Model file for the job. Use its own axes, mm. A direction names the side the tool comes from. Coordinates: 2 decimals unless noted, no trailing zeros. Write each loop counter-clockwise with the first axis right and the second up, starting at its lowest first coordinate (ties: lowest second). Pieces come first, ordered by that corner, then holes. Notation, with made-up numbers: (-16, 42.5) -> (42, 42.5) arc R27 cw to (42, 72.5) -> close; hole circle Ø6 at (-14.75, -26). An arc over 180 degrees is marked (long way). Answer as a JSON object with one key per item and string values. Group by question number.
from build123d import *

# Parameters (mm, degrees)
F1_DEPTH = 50
F1_TAPER = 17
F2_R     = 1
F3_R     = 25
F4_DEPTH = 2


with BuildPart() as f1:
    # F0 (on Top) → F1 (new body)
    with BuildSketch(Plane.XY):
        with BuildLine():
            Line((52.6273290813, 55.3626765174), (-57.3726709187, 55.3626765174))
            ThreePointArc((-57.3726709187, 55.3626765174), (-71.5148065424, 49.5048121412), (-77.3726709187, 35.3626765174))
            Line((-77.3726709187, 35.3626765174), (-77.3726709187, 5.3626765174))
            ThreePointArc((-77.3726709187, 5.3626765174), (-71.5148065424, -8.7794591063), (-57.3726709187, -14.6373234826))
            Line((-57.3726709187, -14.6373234826), (52.6273290813, -14.6373234826))
            ThreePointArc((52.6273290813, -14.6373234826), (66.769464705, -8.7794591063), (72.6273290813, 5.3626765174))
            Line((72.6273290813, 5.3626765174), (72.6273290813, 35.3626765174))
            ThreePointArc((72.6273290813, 35.3626765174), (66.769464705, 49.5048121412), (52.6273290813, 55.3626765174))
        make_face()
    extrude(amount=F1_DEPTH, taper=F1_TAPER)

    # F2
    f2_edges = [f1.edges().sort_by_distance(p)[0] for p in [
        (72.627329, 20.362677, 0),
        (66.769465, 49.504812, 0),
        (-2.372671, 55.362677, 0),
        (-71.514807, 49.504812, 0),
        (-77.372671, 20.362677, 0),
        (-71.514807, -8.779459, 0),
        (-2.372671, -14.637323, 0),
        (66.769465, -8.779459, 0),
        (57.340795, 20.362677, 50),
        (55.960253, 38.6956, 50),
        (-2.372671, 40.076142, 50),
        (-60.705595, 38.6956, 50),
        (-62.086137, 20.362677, 50),
        (-60.705595, 2.029753, 50),
        (-2.372671, 0.649211, 50),
        (55.960253, 2.029753, 50),
    ]]
    fillet(f2_edges, radius=F2_R)

    # F3 (on face) → F4 (cut)
    with BuildSketch(Plane(origin=(0, 0, 0), x_dir=(1, 0, 0), z_dir=(0, 0, -1))):
        with Locations((35.1273290813, -20.0112540795)):
            Circle(F3_R)
        with Locations((-39.8726709187, -20.0112540795)):
            Circle(F3_R)
    extrude(amount=-F4_DEPTH, mode=Mode.SUBTRACT)


solid = f1.part
(1) Cut at A-A on x = -6. List the corners of the cut face in (y, z), plus the area to 3 significant figures.
(2) Pin check, flat tips, straight feed: pin 1 (10 mm diameter, centred on x = -34, z = 17, fed in from +Y); pin 2 (8 mm diameter, centred on y = 6.5, z = 42.5, fed in from -X); pin 3 (4 mm diameter, centred on x = -57.5, z = 19.5, fed in from +Y). Stop position of each tip, or through.
(3) Cut at B-B on z = 19. List the corners of the cut face in (x, y), plus the area to 3 significant figures.
(4) Wall check: probe 1 along Z at (x, y) = (-39, 30); probe 2 along X at (y, z) = (30, 27); probe 3 along X at (y, z) = (41, 25.5). Give the ranges that are in metal, low to high.
(5) Cut at C-C on y = 26.5. List the corners of the cut face in (x, z), plus the area to 3 significant figures.
(6) 3-axis set-ups, long thin cutter, end or side, ignore diameter. For faces 1 (the face through (64.997, 20.573, 24.956)), 2 (the face through (35, 20, 2)): which of +Z, -Z, +X, -X, +Y, -Y reach the whole face in a straight line?
(7) Pull direction X, two halves, no side cores. Call faces 3 (the face through (61.32, 43.87, 25.63)), 4 (the face through (48.567, -1.069, 0.986)), 5 (the face through (-66.07, -3.14, 25.63)): released by +X, released by -X, zero draft, split by the parting line, or undercut.
(8) Cut at D-D on y = 15. List the corners of the cut face in (x, z).
Results found:
{
 "1": {"outline": "(-14.24, 1.29) arc R1 ccw to (-13.29, 0) -> (54.01, 0) arc R1 ccw to (54.97, 1.29) -> (40.29, 49.29) arc R1 ccw to (39.34, 50) -> (1.39, 50) arc R1 ccw to (0.43, 49.29) -> close", "area": "2,730 mm²"},
 "2": {"pin 1": "stops at y = 51.69", "pin 2": "stops at x = -65.6", "pin 3": "stops at y = 50.01"},
 "3": {"outline": "(-71.56, 5.36) arc R14.19 ccw to (-57.37, -8.83) -> (52.63, -8.83) arc R14.19 ccw to (66.82, 5.36) -> (66.82, 35.36) arc R14.19 ccw to (52.63, 49.55) -> (-57.37, 49.55) arc R14.19 ccw to (-71.56, 35.36) -> close", "area": "7,910 mm²"},
 "4": {"probe 1": "z = 2 to 50", "probe 2": "x = -69.12 to 64.37", "probe 3": "x = -68.2 to 63.45"},
 "5": {"outline": "(-76.98, 1.29) arc R1 ccw to (-76.02, 0) -> (-64.02, 0) -> (-64.02, 2) -> (-15.73, 2) -> (-15.73, 0) -> (10.98, 0) -> (10.98, 2) -> (59.27, 2) -> (59.27, 0) -> (71.28, 0) arc R1 ccw to (72.23, 1.29) -> (57.56, 49.29) arc R1 ccw to (56.6, 50) -> (-61.35, 50) arc R1 ccw to (-62.3, 49.29) -> close", "area": "6,540 mm²"},
 "6": {"face 1": "+Z, +X, +Y, -Y", "face 2": "-Z"},
 "7": {"face 3": "released by +X", "face 4": "undercut", "face 5": "released by -X"},
 "8": {"outline": "(-76.98, 1.29) arc R1 ccw to (-76.02, 0) -> (-64.37, 0) -> (-64.37, 2) -> (-15.38, 2) -> (-15.38, 0) -> (10.63, 0) -> (10.63, 2) -> (59.62, 2) -> (59.62, 0) -> (71.28, 0) arc R1 ccw to (72.23, 1.29) -> (57.56, 49.29) arc R1 ccw to (56.6, 50) -> (-61.35, 50) arc R1 ccw to (-62.3, 49.29) -> close"}
}
